Build history of the part. All positions in model axes, mm. A direction names the side the tool comes from. Coordinates: 2 decimals unless noted, no trailing zeros. Loops run counter-clockwise (first coordinate to the right, second up) from the corner with the lowest first, then second, coordinate; pieces in that order, holes last.
Item 1: Cut at B-B (y = 3.5). List the corners of the cut face in (x, z).
Item 2: Cut at C-C (z = 0). List the corners of the cut face in (x, y).
Item 3: 3-axis set-ups, long thin cutter, end or side, ignore diameter. For faces 4 (the face through (-22, 1, 20)), 5 (the face through (0, 13.769, 26)), 6 (the face through (3.06, 1.46, 9.73)): which of +Z, -Z, +X, -X, +Y, -Y reach the whole face in a straight line?
Item 4: Cut at A-A (x = 0). List the corners of the cut face in (y, z).
Item 5: Flat gauge pins, fed straight in: pin 1 (1.1 mm diameter, centred on x = 26.5, z = 4, fed in from -Y); pin 2 (1.2 mm diameter, centred on y = 15.5, z = 27, fed in from +X); pin 3 (5 mm diameter, centred on y = 17, z = 21.5, fed in from -X); pin 4 (1.9 mm diameter, centred on x = 20.93, z = -21.83, fed in from +Y). Where does each tip first touch, or does it go through?
Item 6: Cut at D-D (x = -13). List the corners of the cut face in (y, z), and give its area (3 significant figures).
Item 7: Drill centre lines: line 1 along X through (y, z) = (17.75, -10); line 2 along Y through (x, z) = (-5.5, 8). Where is each one in solid material? Low to high.
Item 8: Mould opens along X. For faces 1 (the face through (0, 0.9, 0)), 2 (the face through (0.25, 0.63, 26.84)), 3 (the face through (-27.5, 13, 0)) say: released by +X, released by -X, zero draft, split by the parting line, or undercut.
from build123d import *

# Parameters (mm, degrees)
EXTRUDE_2_DEPTH      = 25
CUT_EXTRUDE_1_DEPTH  = 23
SKETCH_4_R           = 1.2
CUT_EXTRUDE_2_DEPTH  = 10
SKETCH_5_R           = 2.05
CUT_EXTRUDE_3_DEPTH  = 1
CUT_EXTRUDE_4_DEPTH  = 8
SKETCH_8_W           = 8.296155167
SKETCH_8_H           = 2.779340605
CUT_EXTRUDE_9_DEPTH  = 8
SKETCH_11_R          = 10.2
CUT_EXTRUDE_11_DEPTH = 1.1
FILLET_3_R           = 2.2
FILLET_4_R           = 1


with BuildPart() as part:
    # 草图1 → 凸台-拉伸2 (new body)
    with BuildSketch(Plane(origin=(0, 0, 0), x_dir=(1, 0, 0), z_dir=(0, 1, 0))):
        with BuildLine():
            Line((-17.5, 27.5), (17.5, 27.5))
            ThreePointArc((17.5, 27.5), (24.571067812, 24.571067812), (27.5, 17.5))
            Line((27.5, 17.5), (27.5, -17.5))
            ThreePointArc((27.5, -17.5), (24.571067812, -24.571067812), (17.5, -27.5))
            Line((17.5, -27.5), (-17.5, -27.5))
            ThreePointArc((-17.5, -27.5), (-24.571067812, -24.571067812), (-27.5, -17.5))
            Line((-27.5, -17.5), (-27.5, 17.5))
            ThreePointArc((-27.5, 17.5), (-24.571067812, 24.571067812), (-17.5, 27.5))
        make_face()
    extrude(amount=EXTRUDE_2_DEPTH)

    # 草图3 → 切除-拉伸1 (cut)
    with BuildSketch(Plane(origin=(0, 25, 0), x_dir=(1, 0, 0), z_dir=(0, 1, 0))):
        with BuildLine():
            Line((-20.25, 25.25), (20.25, 25.25))
            ThreePointArc((20.25, 25.25), (23.785533906, 23.785533906), (25.25, 20.25))
            Line((25.25, 20.25), (25.25, -20.25))
            ThreePointArc((25.25, -20.25), (23.785533906, -23.785533906), (20.25, -25.25))
            Line((20.25, -25.25), (-20.25, -25.25))
            ThreePointArc((-20.25, -25.25), (-23.785533906, -23.785533906), (-25.25, -20.25))
            Line((-25.25, -20.25), (-25.25, 20.25))
            ThreePointArc((-25.25, 20.25), (-23.785533906, 23.785533906), (-20.25, 25.25))
        make_face()
    extrude(amount=-CUT_EXTRUDE_1_DEPTH, mode=Mode.SUBTRACT)

    # 草图4 → 切除-拉伸2 (cut)
    with BuildSketch(Plane.XZ):
        with Locations(Location((-21.452692405, 21.308392177, 0), (0, 0, 270))):
            Circle(SKETCH_4_R)
        with Locations(Location((21.308392177, 20.927391415, 0), (0, 0, 270))):
            Circle(SKETCH_4_R)
        with Locations(Location((-21.833693167, -21.452692405, 0), (0, 0, 270))):
            Circle(SKETCH_4_R)
        with Locations(Location((20.927391415, -21.833693167, 0), (0, 0, 270))):
            Circle(SKETCH_4_R)
    extrude(amount=-CUT_EXTRUDE_2_DEPTH, mode=Mode.SUBTRACT)

    # 草图5 → 切除-拉伸3 (cut)
    with BuildSketch(Plane.XZ):
        with Locations(Location((-21.452692405, 21.308392177, 0), (0, 0, 270))):
            Circle(SKETCH_5_R)
        with Locations(Location((21.308392177, 20.927391415, 0), (0, 0, 270))):
            Circle(SKETCH_5_R)
        with Locations(Location((-21.833693167, -21.452692405, 0), (0, 0, 270))):
            Circle(SKETCH_5_R)
        with Locations(Location((20.927391415, -21.833693167, 0), (0, 0, 270))):
            Circle(SKETCH_5_R)
    extrude(amount=-CUT_EXTRUDE_3_DEPTH, mode=Mode.SUBTRACT)

    # 草图7 → 切除-拉伸4 (cut)
    with BuildSketch(Plane.XY.offset(27.5)):
        with BuildLine():
            Line((-3.815614102, 17.230683857), (3.328314128, 17.230683857))
            ThreePointArc((3.328314128, 17.230683857), (4.035420909, 16.937790638), (4.328314128, 16.230683857))
            Line((4.328314128, 16.230683857), (4.328314128, 14.769316156))
            ThreePointArc((4.328314128, 14.769316156), (4.035420909, 14.062209375), (3.328314128, 13.769316156))
            Line((3.328314128, 13.769316156), (-3.815614102, 13.769316156))
            ThreePointArc((-3.815614102, 13.769316156), (-4.522720884, 14.062209375), (-4.815614102, 14.769316156))
            Line((-4.815614102, 14.769316156), (-4.815614102, 16.230683857))
            ThreePointArc((-4.815614102, 16.230683857), (-4.522720884, 16.937790638), (-3.815614102, 17.230683857))
        make_face()
    extrude(amount=-CUT_EXTRUDE_4_DEPTH, mode=Mode.SUBTRACT)

    # 草图8 → 切除-拉伸9 (cut)
    with BuildSketch(Plane(origin=(27.5, 0, 0), x_dir=(0, 0, -1), z_dir=(1, 0, 0))):
        with Locations((-5.725361951, 19.869366797)):
            Rectangle(SKETCH_8_W, SKETCH_8_H)
    extrude(amount=-CUT_EXTRUDE_9_DEPTH, mode=Mode.SUBTRACT)

    # 草图11 → 切除-拉伸11 (cut)
    with BuildSketch(Plane(origin=(0, 2, 0), x_dir=(1, 0, 0), z_dir=(0, 1, 0))):
        with Locations(Location((0, 0, 0), (0, 0, 270))):
            Circle(SKETCH_11_R)
    extrude(amount=-CUT_EXTRUDE_11_DEPTH, mode=Mode.SUBTRACT)

    # 圆角3
    # the kernel refuses this fillet: 2.2 mm, written as the material it takes off along each edge
    with BuildSketch(Plane(origin=(17.5, 0, 27.5), x_dir=(0, 0, -1), z_dir=(-1, 0, 0)), Plane(origin=(-27.5, 0, 17.5), x_dir=(1, 0, 0), z_dir=(0, 0, -1)), Plane(origin=(27.5, 0, -17.5), x_dir=(-1, 0, 0), z_dir=(0, 0, 1))) as fillet_3_piece_1:
        with BuildLine():
            CenterArc((FILLET_3_R, -FILLET_3_R), FILLET_3_R, 90, 90)
            Line((0, -FILLET_3_R), (0, 0))
            Line((0, 0), (FILLET_3_R, 0))
        make_face()
    extrude(amount=35, mode=Mode.SUBTRACT)
    with BuildSketch(Plane(origin=(-17.5, 0, 17.5), x_dir=(0, 0, 1), z_dir=(1, 0, 0))) as fillet_3_piece_2:
        with BuildLine():
            CenterArc((10 - FILLET_3_R, -FILLET_3_R), FILLET_3_R, 0, 90)
            Line((10, -FILLET_3_R), (10, 0))
            Line((10, 0), (10 - FILLET_3_R, 0))
        make_face()
    revolve(axis=Axis((-17.5, 0, 17.5), (0, -1, 0)), revolution_arc=90, mode=Mode.SUBTRACT)
    with BuildSketch(Plane(origin=(-17.5, 0, -17.5), x_dir=(-1, 0, 0), z_dir=(0, 0, 1))) as fillet_3_piece_3:
        with BuildLine():
            CenterArc((10 - FILLET_3_R, -FILLET_3_R), FILLET_3_R, 0, 90)
            Line((10 - FILLET_3_R, 0), (10, 0))
            Line((10, 0), (10, -FILLET_3_R))
        make_face()
    revolve(axis=Axis((-17.5, 0, -17.5), (0, -1, 0)), revolution_arc=90, mode=Mode.SUBTRACT)
    with BuildSketch(Plane(origin=(-17.5, 0, -27.5), x_dir=(0, 1, 0), z_dir=(1, 0, 0))) as fillet_3_piece_4:
        with BuildLine():
            CenterArc((FILLET_3_R, FILLET_3_R), FILLET_3_R, 180, 90)
            Line((0, FILLET_3_R), (0, 0))
            Line((0, 0), (FILLET_3_R, 0))
        make_face()
    extrude(amount=35, mode=Mode.SUBTRACT)
    with BuildSketch(Plane(origin=(17.5, 0, -17.5), x_dir=(0, 0, -1), z_dir=(-1, 0, 0))) as fillet_3_piece_5:
        with BuildLine():
            CenterArc((10 - FILLET_3_R, -FILLET_3_R), FILLET_3_R, 0, 90)
            Line((10 - FILLET_3_R, 0), (10, 0))
            Line((10, 0), (10, -FILLET_3_R))
        make_face()
    revolve(axis=Axis((17.5, 0, -17.5), (0, -1, 0)), revolution_arc=90, mode=Mode.SUBTRACT)
    with BuildSketch(Plane(origin=(17.5, 0, 17.5), x_dir=(1, 0, 0), z_dir=(0, 0, -1))) as fillet_3_piece_6:
        with BuildLine():
            CenterArc((10 - FILLET_3_R, -FILLET_3_R), FILLET_3_R, 0, 90)
            Line((10, -FILLET_3_R), (10, 0))
            Line((10, 0), (10 - FILLET_3_R, 0))
        make_face()
    revolve(axis=Axis((17.5, 0, 17.5), (0, -1, 0)), revolution_arc=90, mode=Mode.SUBTRACT)

    # 圆角4
    fillet_4_edges = [part.edges().sort_by_distance(p)[0] for p in [
        (-24.571067812, 25, 24.571067812),
        (0, 25, 27.5),
        (24.571067812, 25, 24.571067812),
        (27.5, 25, 0),
        (24.571067812, 25, -24.571067812),
        (0, 25, -27.5),
        (-24.571067812, 25, -24.571067812),
        (-27.5, 25, 0),
    ]]
    fillet(fillet_4_edges, radius=FILLET_4_R)


solid = part.part
Filled sheet:
1. outline: (-27.5, -17.5) arc R10 ccw to (-17.5, -27.5) - (17.5, -27.5) arc R10 ccw to (27.5, -17.5) - (27.5, 17.5) arc R10 ccw to (17.5, 27.5) - (-17.5, 27.5) arc R10 ccw to (-27.5, 17.5) - close; hole (-25.25, -20.25) arc R5 ccw to (-20.25, -25.25) - (20.25, -25.25) arc R5 ccw to (25.25, -20.25) - (25.25, 20.25) arc R5 ccw to (20.25, 25.25) - (-20.25, 25.25) arc R5 ccw to (-25.25, 20.25) - close
2. outline: (-27.5, 2.2) arc R2.2 ccw to (-25.3, 0) - (25.3, 0) arc R2.2 ccw to (27.5, 2.2) - (27.5, 24) arc R1 ccw to (26.5, 25) - (25.25, 25) - (25.25, 2) - (10.2, 2) - (10.2, 0.9) - (-10.2, 0.9) - (-10.2, 2) - (-25.25, 2) - (-25.25, 25) - (-26.5, 25) arc R1 ccw to (-27.5, 24) - close
3. face 4: -Y
3. face 5: +Z
3. face 6: +Y
4. outline: (0, -25.3) arc R2.2 ccw to (2.2, -27.5) - (24, -27.5) arc R1 ccw to (25, -26.5) - (25, -25.25) - (2, -25.25) - (2, -10.2) - (0.9, -10.2) - (0.9, 10.2) - (2, 10.2) - (2, 25.25) - (13.77, 25.25) - (13.77, 27.5) - (2.2, 27.5) arc R2.2 ccw to (0, 25.3) - close; (17.23, 25.25) - (25, 25.25) - (25, 26.5) arc R1 ccw to (24, 27.5) - (17.23, 27.5) - close
5. pin 1: stops at y = 0.1
5. pin 2: stops at x = 22.06
5. pin 3: stops at x = -27.39
5. pin 4: passes through
6. outline: (0, -25.3) arc R2.2 ccw to (2.2, -27.5) - (24, -27.5) arc R1 ccw to (25, -26.5) - (25, -25.25) - (2, -25.25) - (2, 25.25) - (25, 25.25) - (25, 26.5) arc R1 ccw to (24, 27.5) - (2.2, 27.5) arc R2.2 ccw to (0, 25.3) - close
6. area: 211 mm2
7. line 1: x = -27.5 to -25.25, 25.25 to 27.5
7. line 2: y = 0 to 0.9
8. face 1: undercut
8. face 2: zero draft
8. face 3: released by -X
